Design review of the part built by this model. Coordinates are the model's own, in mm. Face numbers are marked on the shaded views. A direction names the side the tool comes from. Coordinates: 2 decimals unless noted, no trailing zeros. Loops run counter-clockwise (first coordinate to the right, second up) from the corner with the lowest first, then second, coordinate; pieces in that order, holes last. Notation, with made-up numbers: (60.5, 64.5) - (103.5, 64.5) arc R20 cw to (103.5, 84.5) - close; hole circle Ø1 at (24.5, 81). An arc over 180 degrees is marked (long way). Answer in a Markdown table with one row per item. Add a question column.
(1) Clearance check with flat-ended pins moving along their axes: pin 1 (6 mm diameter, centred on y = 33.5, z = 0, fed in from +X); pin 2 (22.5 mm diameter, centred on x = 9.5, z = -4.5, fed in from +Y); pin 3 (16.5 mm diameter, centred on x = 63.89, z = 15.06, fed in from -Y); pin 4 (4 mm diameter, centred on y = 37, z = -31, fed in from -X). State where each tip first meets the part, or that it passes through.
(2) We need section D-D, the plane y = 41.5. Write out the cut boundary in (x, z) (3 decimals).
(3) We need section C-C, the plane z = 16. Give the number of separate pieces and of enclosed holes in the cut face, plus the area to 3 significant figures.
(4) For the marked faces 1 and 2, list the 3-axis set-ups (+Z, -Z, +X, -X, +Y, -Y) from which the entire face can be reached by the end or side of a thin tool; tool diameter is ignored.
(5) We need section B-B, the plane x = -40.5. Write out the cut boundary in (y, z) (3 decimals).
(6) We need section A-A, the plane y = 6.5. Write out the cut boundary in (x, z), plus the area to 3 significant figures.
(7) To check wall thickness, follow L1, parallel to X at y = 35.5, z = -5; L2, parallel to Z at x = -46, y = 19; L3, parallel to Y at x = 2.5, z = 5.5. State the ranges of each line that lie inside material, in increasing order. Write a range as [from, to].
from build123d import *

# Parameters (mm, degrees)
SKETCH3_W           = 152.4
SKETCH3_H           = 76.2
BOSS_EXTRUDE2_DEPTH = 25.4
SKETCH4_R           = 6.35
CUT_EXTRUDE1_DEPTH  = 97.416192211
SKETCH5_R           = 28.575
BOSS_EXTRUDE3_DEPTH = 19.05
SKETCH6_R           = 22.353274987
CUT_EXTRUDE3_DEPTH  = 18.034
CHAMFER1_SIZE       = 3.175
FILLET1_R           = 6.35


with BuildPart() as part:
    # Sketch3 → Boss-Extrude2 (new body)
    with BuildSketch(Plane(origin=(0, 0, 0), x_dir=(1, 0, 0), z_dir=(0, 1, 0))):
        with Locations((6.742008695, 3.989729317)):
            Rectangle(SKETCH3_W, SKETCH3_H)
    extrude(amount=BOSS_EXTRUDE2_DEPTH)

    # Sketch4 → Cut-Extrude1 (cut, through all)
    with BuildSketch(Plane(origin=(0, 25.4, 0), x_dir=(1, 0, 0), z_dir=(0, 1, 0))):
        with Locations(Location((-50.407991305, 23.039729317, 0), (0, 0, 270))):
            Circle(SKETCH4_R)
        with Locations(Location((-50.407991305, -15.060270683, 0), (0, 0, 270))):
            Circle(SKETCH4_R)
        with Locations(Location((63.892008695, 23.039729317, 0), (0, 0, 270))):
            Circle(SKETCH4_R)
        with Locations(Location((63.892008695, -15.060270683, 0), (0, 0, 270))):
            Circle(SKETCH4_R)
    extrude(amount=-CUT_EXTRUDE1_DEPTH, mode=Mode.SUBTRACT)

    # Sketch5 → Boss-Extrude3 (add)
    with BuildSketch(Plane(origin=(0, 25.4, 0), x_dir=(1, 0, 0), z_dir=(0, 1, 0))):
        with Locations(Location((1.327722903, 3.693056123, 0), (0, 0, 90))):
            Circle(SKETCH5_R)
    extrude(amount=BOSS_EXTRUDE3_DEPTH)

    # Sketch6 → Cut-Extrude3 (cut)
    with BuildSketch(Plane(origin=(0, 44.45, 0), x_dir=(1, 0, 0), z_dir=(0, 1, 0))):
        with Locations(Location((1.440777923, 3.989157158, 0), (0, 0, 270))):
            Circle(SKETCH6_R)
    extrude(amount=-CUT_EXTRUDE3_DEPTH, mode=Mode.SUBTRACT)

    # Chamfer1
    chamfer1_edges = [part.edges().sort_by_distance(p)[0] for p in [
        (82.942008695, 25.4, -3.989729317),
        (6.742008695, 25.4, -42.089729317),
        (-69.457991305, 25.4, -3.989729317),
        (6.742008695, 25.4, 34.110270683),
    ]]
    chamfer(chamfer1_edges, length=CHAMFER1_SIZE)

    # Fillet1
    fillet1_edges = [part.edges().sort_by_distance(p)[0] for p in [
        (1.327722903, 25.4, 24.881943877),
        (-69.457991305, 11.1125, 34.110270683),
        (-69.457991305, 11.1125, -42.089729317),
        (82.942008695, 11.1125, -42.089729317),
        (82.942008695, 11.1125, 34.110270683),
    ]]
    fillet(fillet1_edges, radius=FILLET1_R)


solid = part.part
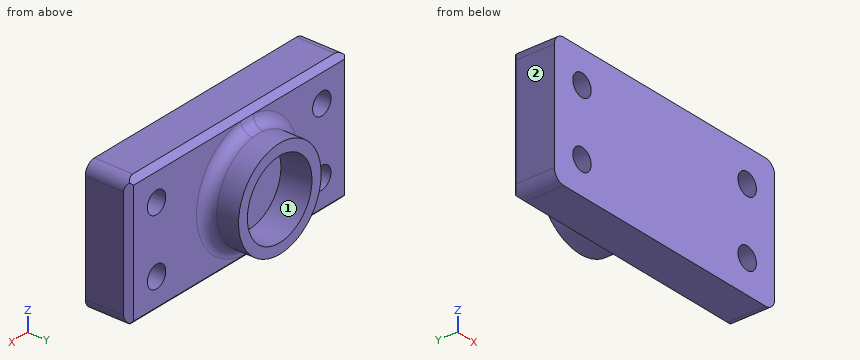
Responses:
| question | item | result |
|---|---|---|
| 1 | pin 1 | stops at x = 29.89 |
| 1 | pin 2 | stops at y = 26.42 |
| 1 | pin 3 | stops at y = 0 |
| 1 | pin 4 | stops at x = -11.94 |
| 2 | outline | circle Ø57.15 at (1.328, -3.693); hole circle Ø44.707 at (1.441, -3.989) |
| 3 | separate pieces | 3 |
| 3 | enclosed holes | 0 |
| 3 | area | 3,670 mm2 |
| 4 | face 1 | +Y |
| 4 | face 2 | +Z, -Z, -X, +Y, -Y |
| 5 | outline | (0, -42.09) - (22.225, -42.09) - (25.4, -38.915) - (25.4, 30.935) - (22.225, 34.11) - (0, 34.11) - close |
| 6 | outline | (-69.46, -35.74) arc R6.35 ccw to (-63.11, -42.09) - (76.59, -42.09) arc R6.35 ccw to (82.94, -35.74) - (82.94, 27.76) arc R6.35 ccw to (76.59, 34.11) - (-63.11, 34.11) arc R6.35 ccw to (-69.46, 27.76) - close; hole circle Ø12.7 at (-50.41, -23.04); hole circle Ø12.7 at (-50.41, 15.06); hole circle Ø12.7 at (63.89, -23.04); hole circle Ø12.7 at (63.89, 15.06) |
| 6 | area | 11,100 mm2 |
| 7 | L1 | x = [-27.22, -20.89], [23.77, 29.87] |
| 7 | L2 | z = [-42.09, -27.61], [-18.47, 10.49], [19.63, 34.11] |
| 7 | L3 | y = [0, 26.42] |
